from build123d import *

# Parameters (mm, degrees)
F0_W     = 101.6
F0_H     = 101.6
F1_DEPTH = 6.35
F2_W     = 6.35
F2_H     = 76.2
F3_DEPTH = 107.95
F4_R     = 6.35
F5_DEPTH = 82.551
F6_SIZE  = 12.7


with BuildPart() as f1:
    # F0 (on Top) → F1 (new body)
    with BuildSketch(Plane.XY):
        with Locations((-21.764829, -22.656878)):
            Rectangle(F0_W, F0_H)
    extrude(amount=F1_DEPTH)

    # F2 (on face) → F3 (join)
    with BuildSketch(Plane.XY.offset(6.35)):
        with Locations((-50.339829, -22.656878)):
            Rectangle(F2_W, F2_H)
        with Locations((6.810171, -22.656878)):
            Rectangle(F2_W, F2_H)
    extrude(amount=F3_DEPTH)

    # F4 (on face) → F5 (cut, through all)
    with BuildSketch(Plane.YZ.offset(9.985171)):
        with Locations((-22.656878, 88.9)):
            Circle(F4_R)
    extrude(amount=-F5_DEPTH, mode=Mode.SUBTRACT)

    # F6
    f6_edges = [f1.edges().sort_by_distance(p)[0] for p in [
        (6.810171, -60.756878, 114.3),
        (6.810171, 15.443122, 114.3),
        (-50.339829, -60.756878, 114.3),
        (-50.339829, 15.443122, 114.3),
    ]]
    chamfer(f6_edges, length=F6_SIZE)


solid = f1.part
Read the model definition and answer for the solid it produces. Units are mm, in the model's axes. A direction names the side the tool comes from. Give positions to 0.01 mm unless a question says otherwise; leave off trailing zeros. Write each loop counter-clockwise with the first axis right and the second up, starting at its lowest first coordinate (ties: lowest second). Pieces come first, ordered by that corner, then holes. Notation, with made-up numbers: (17, 66) - (29, 66) arc R17 ccw to (29, 71) - close; hole circle Ø8 at (86, 22). An arc over 180 degrees is marked (long way). Use CSV: the item, a comma, the result in double quotes. Start each with the question number.
Item 1: Consider line 1 (X direction, y = 13, z = 8); line 2 (Z direction, x = -25, y = -50.5); line 3 (Y direction, x = -48, z = 88). Determine where each line is inside the solid, lowest interval first.
Item 2: Flat-ended cylindrical pins translate along their axes: P1, Ø8, axis at y = -6.5, z = 76.5, coming from the +X side; P2, Ø23, axis at y = -30, z = 71.5, coming from the -X side; P3, Ø3, axis at x = 7.5, z = 33.5, coming from the +Y side; P4, Ø6, axis at x = -59.5, z = 22.5, coming from the -Y side. Find the tip coordinate at first contact, or state that the pin passes through.
Item 3: The part is cut by section B-B, the plane z = 88.9. Give the vertices of the cut face in (x, y).
Item 4: The part is cut by section C-C, the plane y = -44. Give the vertices of the cut face in (x, z).
Item 5: The part is cut by section A-A, the plane z = 52. Give the vertices of the cut face in (x, y), and give its area (3 significant figures).
Item 6: For faces 1 (the flat face through (-53.515, -23, 60)), 2 (the flat face through (7, -60.757, 53)), 3 (the flat face through (-50, 15.443, 53)), determine the directions among +Z, -Z, +X, -X, +Y, -Y from which every point of the face is accessible in a straight line to the end or side of a thin tool.
Item 7: The part is cut by section D-D, the plane x = -32. Give the vertices of the cut face in (y, z), and give its area (3 significant figures).
Item 8: The mould has two halves that part along X. Classify faces 4 (the flat face through (6.766, 9.004, 108.039)), 5 (the flat face through (9.985, -23, 60)), 6 (the flat face through (-22, -22, 6.35)): pulls with the +X half, pulls with the -X half, needs draft (parallel to the pull), parting line crosses it, or undercut.
Taken from the geometry:
1,line 1,"-53.51 to -47.16, 3.64 to 9.99"
1,line 2,"0 to 6.35"
1,line 3,"-60.76 to -28.94, -16.37 to 15.44"
2,P1,"x = 9.99"
2,P2,"x = -53.51"
2,P3,"y = 15.44"
2,P4,"through"
3,outline,"(-53.51, -60.76) - (-47.16, -60.76) - (-47.16, -29.01) - (-53.51, -29.01) - close; (-53.51, -16.31) - (-47.16, -16.31) - (-47.16, 15.44) - (-53.51, 15.44) - close; (3.64, -60.76) - (9.99, -60.76) - (9.99, -29.01) - (3.64, -29.01) - close; (3.64, -16.31) - (9.99, -16.31) - (9.99, 15.44) - (3.64, 15.44) - close"
4,outline,"(-72.56, 0) - (29.04, 0) - (29.04, 6.35) - (9.99, 6.35) - (9.99, 114.3) - (3.64, 114.3) - (3.64, 6.35) - (-47.16, 6.35) - (-47.16, 114.3) - (-53.51, 114.3) - (-53.51, 6.35) - (-72.56, 6.35) - close"
5,outline,"(-53.51, -60.76) - (-47.16, -60.76) - (-47.16, 15.44) - (-53.51, 15.44) - close; (3.64, -60.76) - (9.99, -60.76) - (9.99, 15.44) - (3.64, 15.44) - close"
5,area,"968 mm2"
6,face 1,"+Z, -X, +Y, -Y"
6,face 2,"+Z, +X, -X, -Y"
6,face 3,"+Z, +X, -X, +Y"
7,outline,"(-73.46, 0) - (28.14, 0) - (28.14, 6.35) - (-73.46, 6.35) - close"
7,area,"645 mm2"
8,face 4,"needs draft"
8,face 5,"pulls with the +X half"
8,face 6,"undercut"
